The figure shows three views and two pictorial views of one solid part (mm, origin at its lowest corner). Answer the questions. A direction names the side the tool comes from. Coordinates: 2 decimals unless noted, no trailing zeros. Write each loop counter-clockwise with the first axis right and the second up, starting at its lowest first coordinate (ties: lowest second). Pieces come first, ordered by that corner, then holes. Notation, with made-up numbers: M -29,64.5 L -6,64.5 A16 cw -6,71.5 Z; hole C 26.25,51 d6. An arc over 180 degrees is marked long. Write item = value, one per line.
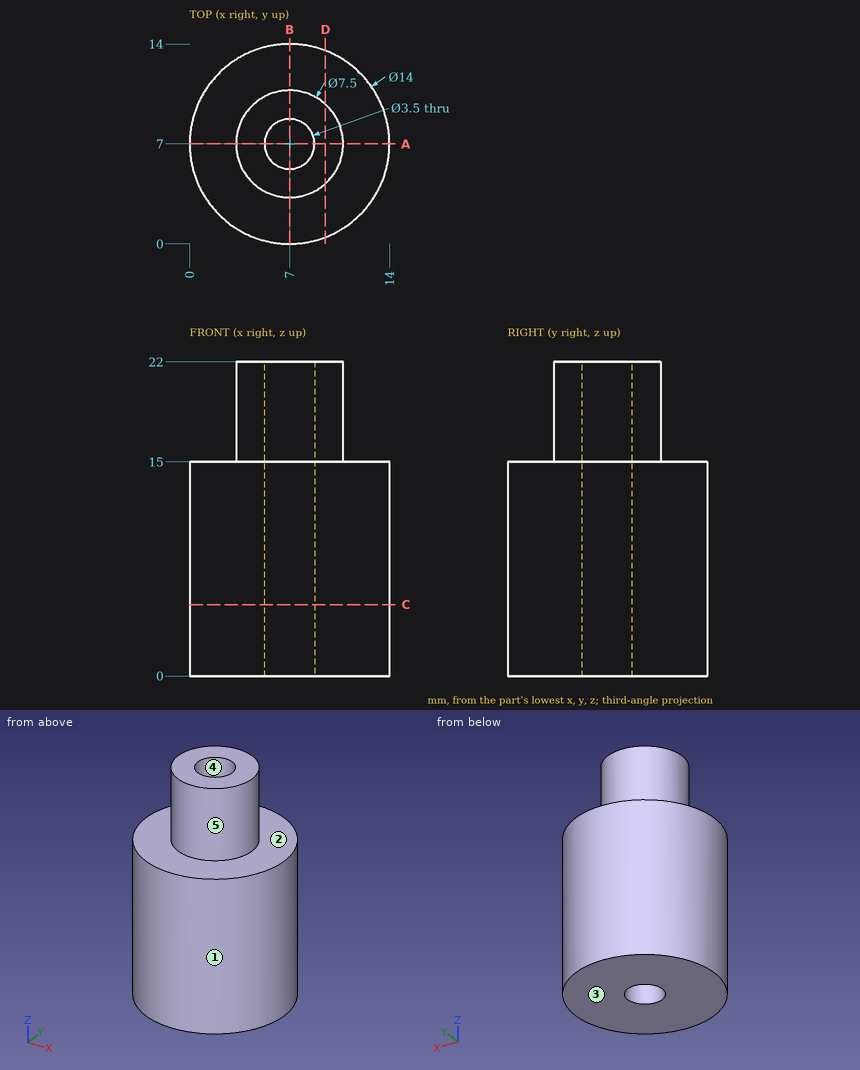
Item 1: For a pull along X with two mould halves and no side action, classify the marked faces 3, 4 and 5 as released by +X, released by -X, zero draft, split by the parting line, or undercut.
Worked answers:
face_3 = zero draft
face_4 = undercut
face_5 = split by the parting line
Item 2: Flat-ended cylindrical pins translate along their axes: pin 1 (3 mm diameter, centred on x = 7, y = 7, fed in from -Z); pin 2 (1.5 mm diameter, centred on y = 11.5, z = 7.5, fed in from -X); pin 3 (8 mm diameter, centred on x = 12, z = 6, fed in from -Y); pin 4 (6 mm diameter, centred on y = 2.5, z = 15.5, fed in from -X). Find the tip coordinate at first contact, or state that the pin passes through.
Worked answers:
pin_1 = through
pin_2 = 1.09
pin_3 = 0.07
pin_4 = 0.17
Item 3: Find section C-C (z = 5). Determine the outline of the cut face in (x, y).
Worked answers:
outline = C 7,7 d14; hole C 7,7 d3.5
Item 4: Find section D-D (x = 9.5). Determine the outline of the cut face in (y, z).
Worked answers:
outline = M 0.46,0 L 13.54,0 L 13.54,15 L 9.8,15 L 9.8,22 L 4.2,22 L 4.2,15 L 0.46,15 Z
Item 5: Find section A-A (y = 7). Determine the outline of the cut face in (x, z), and give its area (4 significant figures).
Worked answers:
outline = M 0,0 L 5.25,0 L 5.25,22 L 3.25,22 L 3.25,15 L 0,15 Z; M 8.75,0 L 14,0 L 14,15 L 10.75,15 L 10.75,22 L 8.75,22 Z
area = 185.5 mm²
Item 6: Which of the six approach directions +Z, -Z, +X, -X, +Y, -Y give full straight-line access (tool end or side, diameter ignored) to the marked faces 1 and 2?
Worked answers:
face_1 = +Z, -Z
face_2 = +Z
Item 7: Consider line 1 along Y through (x, z) = (7, 7.75); line 2 along Z through (x, y) = (5.5, 11); line 3 along Y through (x, z) = (8.25, 3.75). Determine where each line is inside the solid, lowest interval first. Write a range as from..to.
Worked answers:
line_1 = 0..5.25, 8.75..14
line_2 = 0..15
line_3 = 0.11..5.78, 8.22..13.89
